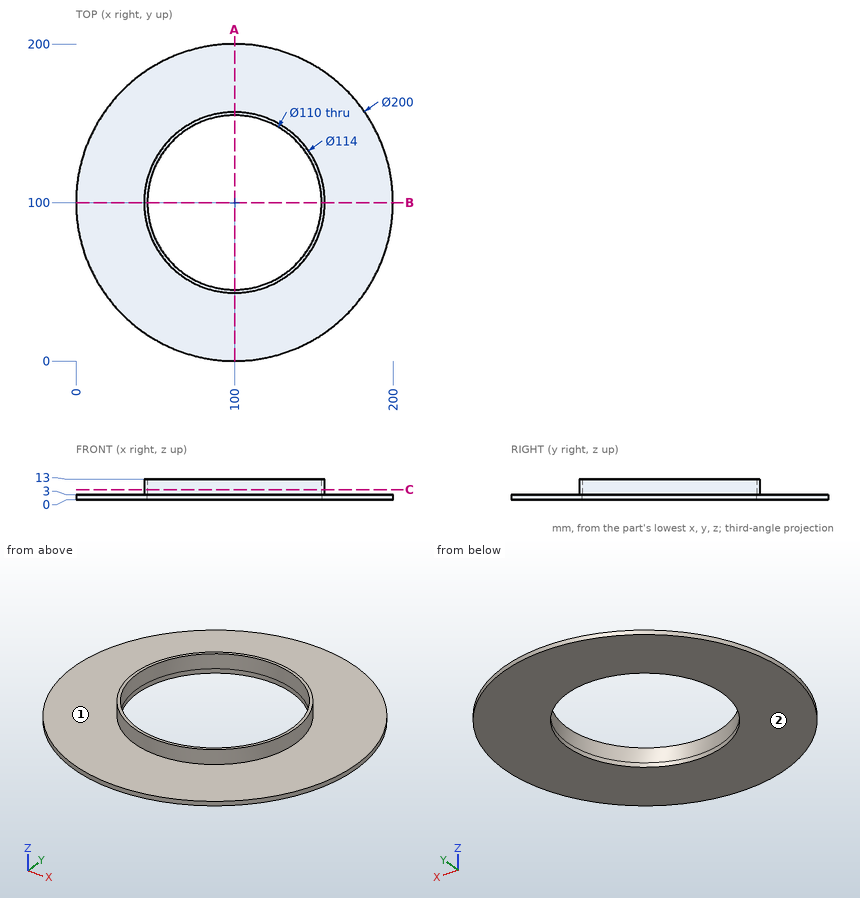
Geometry check sheet. Reference: drawing and pictorial views, mm from the part's lowest x, y, z. A direction names the side the tool comes from. Give positions to 0.01 mm unless a question says otherwise; leave off trailing zeros. Order: outer loops, then holes, each group sorted by start corner. A loop starts at its lowest first (then second) coordinate and runs counter-clockwise, first axis right, second up. Notation, with made-up numbers: M -4.5,25.5 L 34.5,25.5 A15 ccw 34.5,48.5 Z; hole C 60,48 d1. An arc over 180 degrees is marked long. Return JSON: item names as keys, results as strings. Group by question number.
1) Access from +Z, -Z, +X, -X, +Y, -Y to the whole of each face (thin tool, end or side, straight path). Record for the marked faces 1 and 2.
2) Go/stop test with flat-tipped pins: pin 1 Ø5 at (x, z) = (132, 9.5) entering from +Y; pin 2 Ø2 at (x, z) = (174, 2) entering from +Y; pin 3 Ø10 at (x, y) = (56, 55) entering from -Z. Record where each tip stops, or that it passes through.
3) Section check A-A on x = 100. Record the cut outline in (y, z).
4) Section check C-C on z = 6.25. Record the cut outline in (x, y), and give its area (3 significant figures).
5) Scan lines: line 1 (Y direction, x = 100, z = 0.95); line 2 (Z direction, x = 175, y = 142); line 3 (Y direction, x = 73, z = 12). Record each from-to range of solid material in increasing order.
Answer block:
{
 "1": {"face 1": "+Z", "face 2": "-Z, +X, -X, +Y, -Y"},
 "2": {"pin 1": "stops at y = 148.77", "pin 2": "stops at y = 168.34", "pin 3": "stops at z = 0"},
 "3": {"outline": "M 0,0 L 45,0 L 45,13 L 43,13 L 43,3 L 0,3 Z; M 155,0 L 200,0 L 200,3 L 157,3 L 157,13 L 155,13 Z"},
 "4": {"outline": "C 100,100 d114; hole C 100,100 d110", "area": "704 mm^2"},
 "5": {"line 1": "y = 0 to 45, 155 to 200", "line 2": "z = 0 to 3", "line 3": "y = 49.8 to 52.08, 147.92 to 150.2"}
}
